Part model, mm, in its own coordinate system. A direction names the side the tool comes from. Coordinates: 2 decimals unless noted, no trailing zeros. Write each loop counter-clockwise with the first axis right and the second up, starting at its lowest first coordinate (ties: lowest second). Pieces come first, ordered by that corner, then holes. Notation, with made-up numbers: (-22.75, 63.5) - (24.25, 63.5) arc R24 ccw to (24.25, 81.5) - close; hole circle Ø1 at (-11.5, -37.75). An arc over 180 degrees is marked (long way). Use one line per item in the form item = value. Start each with the question number.
Autodesk Inventor part; units mm, degrees
ref_plane "作業平面1" through (0, 0, 0) normal (1, 0, 0) x (0, 0.3162, -0.9487)
ref_plane "YZ Plane" through (0, 0, 0) normal (1, 0, 0) x (0, 1, 0)
ref_plane "XZ Plane" through (0, 0, 0) normal (0, 1, 0) x (-1, 0, 0)
sketch "スケッチ1" plane through (0, 0, 0) normal (0, 0, 1) x (1, 0, 0)
  circle A0 centre (0, 0) radius 18.5
  dimension "d0" = 37
extrude "押し出し1" add sketch "スケッチ1" along normal blind 25
sketch "スケッチ2" plane through (0, 0, 25) normal (0, 0, 1) x (1, 0, 0)
  circle A0 centre (0, 0) radius 18
  dimension "d3" = 36
extrude "押し出し2" add sketch "スケッチ2" along normal blind 54.5
sketch "スケッチ3" plane through (0, 0, 0) normal (0, 0, -1) x (-1, 0, 0)
  circle A0 centre (0, 0) radius 18.5
  circle A1 centre (0, 7) radius 6
  dimension "d6" = 12
  dimension "d7" = 7
extrude "押し出し3" add sketch "スケッチ3" along normal blind 6 contours A1
sketch "スケッチ4" plane through (0, 7, -6) normal (0, 0, -1) x (-1, 0, 0)
  circle A0 centre (0, 0) radius 3
  point P0 (0, -7)
  dimension "d10" = 6
extrude "押し出し4" add sketch "スケッチ4" along normal blind 15
sketch "スケッチ5" plane through (0, 0, 0) normal (0, 0, -1) x (-1, 0, 0)
  circle A0 centre (0, 0) radius 18.5
  circle A1 centre (0, 0) radius 15.5
  line L0 (0, 0) -> (-15.5, 0)
  line L1 (7.75, 13.4234) -> (0, 0)
  line L2 (0, 0) -> (7.75, -13.4234)
  point P0 (-15.5, 0)
  point P1 (7.75, -13.4234)
  dimension "d13" = 31
  dimension "d14" = 120
  dimension "d15" = 120
hole "Hole1" at (15.5, 0, 0) at (-7.75, -13.4234, 0) at (-7.75, 13.4234, 0) direction (0, 0, 1) diameter 3 depth 3 tip angle 118
ref_plane "作業平面1" through (0, 0, 0) normal (1, 0, 0) x (0, 0.3162, -0.9487)
sketch "スケッチ7" plane through (0, 7, -21) normal (0, 0, -1) x (-1, 0, 0)
  line L0 (1.6583, -2.5) -> (-1.6583, -2.5)
  circle A0 centre (0, 0) radius 3
  point P0 (0, -7)
  dimension "d33" = 2.5
extrude "押し出し5" cut sketch "スケッチ7" against normal blind 12 contours A0 L0 picked at (0.3442, -2.6056)
properties part number "rs380ph_36" material "Steel"
Q1. Pin check, flat tips, straight feed: P1, Ø6, axis at x = 1, y = 10, coming from the -Z side; P2, Ø2.5, axis at x = 1, z = -12.5, coming from the -Y side; P3, Ø12, axis at x = -1, z = 9.5, coming from the -Y side; P4, Ø1, axis at x = 1, y = 12, coming from the -Z side. Stop position of each tip, or through.
Q2. Slice it at B-B (y = 16.5). List the corners of the cut face in (x, z), plus the area to 3 significant figures.
Q3. Slice it at A-A (x = 0). List the corners of the cut face in (y, z).
Q4. Which spindle directions (+Z, -Z, +X, -X, +Y, -Y) get a long thin tool onto all of the face, cutting with end or side? Do faces 1 (the flat face through (0, 4.5, -15)), 2 (the cylindrical face through (17, 0, 2)), 3 (the flat face through (4.02, -17.73, 25)). Say none if no direction does.
Q5. Slice it at C-C (z = 36.5). List the corners of the cut face in (x, y), plus the area to 3 significant figures.
Q6. Mould opens along X. For faces 4 (the cylindrical face through (-2.343, -17.847, 51.868)), 5 (the cylindrical face through (-6.837, -14.614, 1.521)), 6 (the flat face through (0, 0, 79.5)) say: released by +X, released by -X, zero draft, split by the parting line, or undercut.
Q7. Slice it at D-D (x = 7.5). List the corners of the cut face in (y, z), plus the area to 3 significant figures.
Q8. Drill centre lines: probe 1 along Y at (x, z) = (-7.75, 1); probe 2 along Y at (x, z) = (-7, 1); probe 3 along Z at (x, y) = (8, -15). Where is each one in solid material? Low to high.
Solution:
q1.P1 = -21
q1.P2 = 4.5
q1.P3 = -18.5
q1.P4 = -6
q2.outline = (-8.37, 0) - (8.37, 0) - (8.37, 25) - (7.19, 25) - (7.19, 79.5) - (-7.19, 79.5) - (-7.19, 25) - (-8.37, 25) - close
q2.area = 1,200 mm2
q3.outline = (-18.5, 0) - (1, 0) - (1, -6) - (4, -6) - (4, -9) - (4.5, -9) - (4.5, -21) - (10, -21) - (10, -6) - (13, -6) - (13, 0) - (18.5, 0) - (18.5, 25) - (18, 25) - (18, 79.5) - (-18, 79.5) - (-18, 25) - (-18.5, 25) - close
q4.face_1 = -Z, +X, -X, -Y
q4.face_2 = -Z
q4.face_3 = +Z
q5.outline = circle Ø36 at (0, 0)
q5.area = 1,020 mm2
q6.face_4 = split by the parting line
q6.face_5 = undercut
q6.face_6 = zero draft
q7.outline = (-16.91, 0) - (16.91, 0) - (16.91, 25) - (16.36, 25) - (16.36, 79.5) - (-16.36, 79.5) - (-16.36, 25) - (-16.91, 25) - close
q7.area = 2,630 mm2
q8.probe_1 = -16.8 to -14.92, -11.92 to 11.92, 14.92 to 16.8
q8.probe_2 = -17.12 to -14.72, -12.12 to 12.12, 14.72 to 17.12
q8.probe_3 = 0 to 79.5
